from build123d import *

# Parameters (mm, degrees)
F3_DEPTH = 12.7
F5_DEPTH = 1.5875
F7_DEPTH = 12.7


with BuildPart() as f1:
    # F0 (on Top) → F1 (revolve)
    with BuildSketch(Plane.XY):
        with BuildLine():
            Line((-101.6, 0), (0, 0))
            Line((0, 0), (0, 6.35))
            Line((0, 6.35), (-1.0414, 6.35))
            Line((-1.0414, 6.35), (-1.0414, 4.191))
            ThreePointArc((-1.0414, 4.191), (-1.152992, 3.921592), (-1.4224, 3.81))
            Line((-1.4224, 3.81), (-9.251272, 3.81))
            ThreePointArc((-9.251272, 3.81), (-10.466292, 4.051682), (-11.496336, 4.739936))
            Line((-11.496336, 4.739936), (-13.1064, 6.35))
            Line((-13.1064, 6.35), (-101.6, 6.35))
            Line((-101.6, 6.35), (-101.6, 0))
        make_face()
    revolve(axis=Axis((-50.8, 0, 0), (1, 0, 0)))

    # F2 (on Front) → F3 (cut, symmetric)
    with BuildSketch(Plane.XZ):
        Polygon((-1.5875, 0), (0, 0), (0, 6.35), (-12.586023, 6.35), align=None)
    extrude(amount=F3_DEPTH, both=True, mode=Mode.SUBTRACT)

    # F4 (on face) → F5 (cut)
    with BuildSketch(Plane.YZ):
        with BuildLine():
            Line((-6.604, 0), (-6.604, -6.604))
            Line((-6.604, -6.604), (6.35, -6.604))
            Line((6.35, -6.604), (6.35, 0))
            Line((6.35, 0), (6.327862, -0.253033))
            Line((6.327862, -0.253033), (6.096889, -1.115039))
            ThreePointArc((6.096889, -1.115039), (5.733909, -1.776663), (5.106439, -2.195926))
            Line((5.106439, -2.195926), (1.303097, -3.580229))
            ThreePointArc((1.303097, -3.580229), (-2.185326, -3.120969), (-3.81, 0))
            Line((-3.81, 0), (-6.604, 0))
        make_face()
    extrude(amount=-F5_DEPTH, mode=Mode.SUBTRACT)

    # F6 (on Front) → F7 (cut, symmetric)
    with BuildSketch(Plane.XZ):
        Polygon((0, -4.24096), (0, 0), (-0.747796, -4.24096), align=None)
    extrude(amount=F7_DEPTH, both=True, mode=Mode.SUBTRACT)


solid = f1.part
For this review, take the finished solid that the model builds, in its own axes (mm). A direction names the side the tool comes from. Coordinates: 2 decimals unless noted, no trailing zeros. Order: outer loops, then holes, each group sorted by start corner. A loop starts at its lowest first (then second) coordinate and runs counter-clockwise, first axis right, second up. Notation, with made-up numbers: (87.25, -21.5) - (98.25, -21.5) arc R26 ccw to (98.25, 12.5) - close; hole circle Ø11 at (33.25, 82). An arc over 180 degrees is marked (long way). Use one line per item in the form item = value.
Q1. For probe 1 along Z at (x, y) = (-50, 0.5); probe 2 along X at (y, z) = (-0.25, -1); probe 3 along X at (y, z) = (3.75, 4.25), list the stretches that pass through material, from the lowest coordinate up. Write a range as from..to.
Checked values:
probe_1 = -6.33..6.33
probe_2 = -101.6..-0.18
probe_3 = -101.6..-12.42
Q2. For faces 1 (the flat face through (-0.257, 1.199, -1.455)), 2 (the flat face through (-1, 1, 0)), list the 3-axis set-ups (+Z, -Z, +X, -X, +Y, -Y) from which the entire face can be reached by the end or side of a thin tool; tool diameter is ignored.
Checked values:
face_1 = -Z, +X, +Y, -Y
face_2 = +Z, +X, +Y, -Y
Q3. Draft analysis for pull direction Z (two halves, no side actions). For faces 3 (the flat face through (-4.2, -0.05, 1.51)), 4 (the cylindrical face through (-57.97, -1.38, -6.2)), 5 (the flat face through (-1.041, 5, -1)), state which applies: +Z half, -Z half, draft (parallel to the pull), parting line (faces both ways), or undercut.
Checked values:
face_3 = +Z half
face_4 = parting line
face_5 = draft
Q4. Consider section A-A (x = -82). Give the boundary of the cut face in (y, z).
Checked values:
outline = circle Ø12.7 at (0, 0)
Q5. For P1, Ø0.8, axis at x = -1, y = 3, coming from the +Z side; P2, Ø1.5, axis at x = -17, y = -4, coming from the +Z side; P3, Ø6, axis at x = -16.5, z = -4.5, coming from the +Y side, all flat-tipped, find the tip position at first contact; note any pin that passes through.
Checked values:
P1 = 0
P2 = 5.46
P3 = 6.17
